Can you work these out from the model? Positions are in its coordinate system, mm. A direction names the side the tool comes from. Round coordinates to 2 decimals unless told otherwise and drop trailing zeros. Order: outer loops, then holes, each group sorted by start corner. A loop starts at its lowest first (then second) coordinate and runs counter-clockwise, first axis right, second up.
Q1. If I drill on line 1 (Y direction, x = 0, z = 21.9); line 2 (X direction, y = 18.5, z = 0.5); line 3 (Y direction, x = -5.5, z = 10), over which ranges is the centre line in solid material (lowest first)?
Q2. We'd pull the mould along Y, two halves only. Please class faces 1 (the face through (-1.6, 100, -20.1)), 2 (the face through (21.24, 73.735, 0.806)), 3 (the face through (0.751, 4.93, -5.885)): pulls with the +Y half, pulls with the -Y half, needs draft (parallel to the pull), parting line crosses it, or undercut.
Q3. If we section it at B-B (y = 75): Please give me the cut outline in (x, z), plus the area to 3 significant figures.
Q4. If we section it at C-C (x = -13.5): Please give me the cut outline in (y, z), plus the area to 3 significant figures.
Q5. If we section it at D-D (y = 9): Please give me the cut outline in (x, z).
Q6. Will these pins go through, and if not, where does the flat tip stop? P1, Ø12, axis at x = 8.5, z = 5.5, coming from the +Y side; P2, Ø3, axis at y = 26.5, z = 13, coming from the -X side; P3, Ø4, axis at y = 33.5, z = -9.5, coming from the -X side.
Q7. For faces 4 (the face through (0, 10, 0)), 5 (the face through (0.195, 26.487, -21.24)), which set-ups out of +Z, -Z, +X, -X, +Y, -Y let a thin tool reach every point of the face, with its end or its side?
Q8. If we section it at A-A (z = 0): Count the separate pieces of the cut face and the enclosed holes in it, plus the area to 3 significant figures.
from build123d import *

# Parameters (mm, degrees)
SKETCH1_R                             = 22.5
BOSS_EXTRUDE1_DEPTH                   = 100
TAP_DRILL_FOR_M6X1_0_TAP4_D           = 3
TAP_DRILL_FOR_M6X1_0_TAP5_D           = 3
TAP_DRILL_FOR_M6X1_0_TAP6_D           = 3
TAP_DRILL_FOR_M6X1_0_TAP6_ON_FACE_2_D = 3
TAP_DRILL_FOR_M6X1_0_TAP7_D           = 3
TAP_DRILL_FOR_M6X1_0_TAP7_ON_FACE_2_D = 3
SKETCH12_R                            = 20
CUT_EXTRUDE1_DEPTH                    = 90
SKETCH15_R                            = 2.5
CUT_EXTRUDE2_DEPTH                    = 90


with BuildPart() as part:
    # Sketch1 → Boss-Extrude1 (new body)
    with BuildSketch(Plane(origin=(0, 0, 0), x_dir=(1, 0, 0), z_dir=(0, 1, 0))):
        with Locations(Location((0, 0, 0), (0, 0, 270))):
            Circle(SKETCH1_R)
    extrude(amount=BOSS_EXTRUDE1_DEPTH)

    # Tap Drill for M6x1.0 Tap4 (through all)
    with Locations(Plane(origin=(0, 25, 22.5), x_dir=(1, 0, 0), z_dir=(0, 0, 1))):
        with Locations((0, 0)):
            Hole(TAP_DRILL_FOR_M6X1_0_TAP4_D / 2)

    # Tap Drill for M6x1.0 Tap5 (through all)
    with Locations(Plane(origin=(-22.5, 25, 0), x_dir=(0, 0, -1), z_dir=(-1, 0, 0))):
        with Locations((0, 0)):
            Hole(TAP_DRILL_FOR_M6X1_0_TAP5_D / 2)

    # Tap Drill for M6x1.0 Tap6 (through all)
    with Locations(Plane(origin=(-22.5, 50, 0), x_dir=(0, 0, -1), z_dir=(-1, 0, 0))):
        with Locations((0, 0)):
            Hole(TAP_DRILL_FOR_M6X1_0_TAP6_D / 2)

    # Tap Drill for M6x1.0 Tap6 on face 2 (through all)
    with Locations(Plane(origin=(0, 50, 22.5), x_dir=(1, 0, 0), z_dir=(0, 0, 1))):
        with Locations((0, 0)):
            Hole(TAP_DRILL_FOR_M6X1_0_TAP6_ON_FACE_2_D / 2)

    # Tap Drill for M6x1.0 Tap7 (through all)
    with Locations(Plane(origin=(0, 75, 22.5), x_dir=(1, 0, 0), z_dir=(0, 0, 1))):
        with Locations((0, 0)):
            Hole(TAP_DRILL_FOR_M6X1_0_TAP7_D / 2)

    # Tap Drill for M6x1.0 Tap7 on face 2 (through all)
    with Locations(Plane(origin=(-22.5, 75, 0), x_dir=(0, 0, -1), z_dir=(-1, 0, 0))):
        with Locations((0, 0)):
            Hole(TAP_DRILL_FOR_M6X1_0_TAP7_ON_FACE_2_D / 2)

    # Sketch12 → Cut-Extrude1 (cut)
    with BuildSketch(Plane(origin=(0, 100, 0), x_dir=(1, 0, 0), z_dir=(0, 1, 0))):
        with Locations(Location((0, 0, 0), (0, 0, 270))):
            Circle(SKETCH12_R)
    extrude(amount=-CUT_EXTRUDE1_DEPTH, mode=Mode.SUBTRACT)

    # Sketch15 → Cut-Extrude2 (cut)
    with BuildSketch(Plane.XZ):
        with Locations(Location((0, -3.5, 0), (0, 0, 270))):
            Circle(SKETCH15_R)
        with Locations(Location((0, 11.5, 0), (0, 0, 270))):
            Circle(SKETCH15_R)
    extrude(amount=-CUT_EXTRUDE2_DEPTH, mode=Mode.SUBTRACT)


solid = part.part
Solution:
1. line 1: y = 0 to 23.5, 26.5 to 48.5, 51.5 to 73.5, 76.5 to 100
1. line 2: x = -22.49 to -19.99, 19.99 to 22.49
1. line 3: y = 0 to 10
2. face 1: pulls with the +Y half
2. face 2: undercut
2. face 3: needs draft
3. outline: (-22.45, -1.5) arc R22.5 ccw to (-1.5, -22.45) - (-1.5, -19.94) arc R20 cw to (-19.94, -1.5) - close; (-22.45, 1.5) - (-19.94, 1.5) arc R20 cw to (-1.5, 19.94) - (-1.5, 22.45) arc R22.5 ccw to start; (1.5, -22.45) arc R22.5 ccw to (22.45, -1.5) - (19.94, -1.5) arc R20 cw to (1.5, -19.94) - close; (1.5, 19.94) arc R20 cw to (19.94, 1.5) - (22.45, 1.5) arc R22.5 ccw to (1.5, 22.45) - close
3. area: 304 mm2
4. outline: (0, -18) - (100, -18) - (100, -14.76) - (10, -14.76) - (10, 14.76) - (100, 14.76) - (100, 18) - (0, 18) - close
4. area: 944 mm2
5. outline: circle Ø45 at (0, 0); hole circle Ø5 at (0, -3.5); hole circle Ø5 at (0, 11.5)
6. P1: stops at y = 10
6. P2: stops at x = -19.34
6. P3: stops at x = -21.21
7. face 4: +Y
7. face 5: +Z, -Z
8. separate pieces: 7
8. enclosed holes: 0
8. area: 855 mm2
